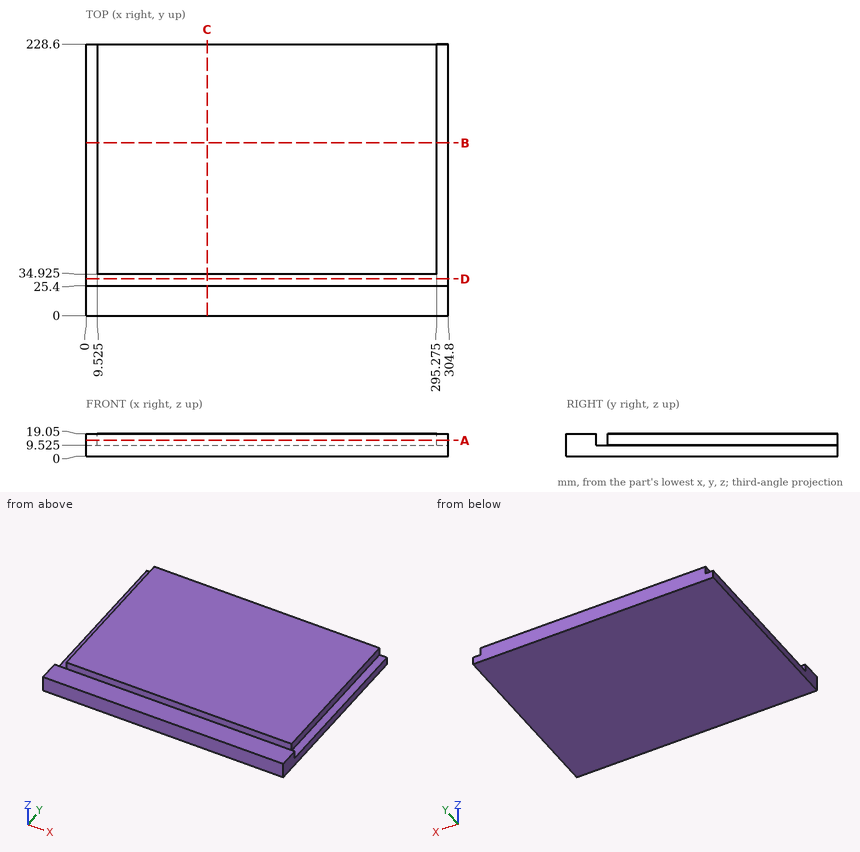
Verification items for this drawing (mm, ordinates from the low corner). Coordinates: 2 decimals unless noted, no trailing zeros. Order: outer loops, then holes, each group sorted by start corner. A loop starts at its lowest first (then second) coordinate and runs counter-clockwise, first axis right, second up. Notation, with made-up numbers: (-29, 44.25) -> (-4, 44.25) arc R23 cw to (-4, 74.25) -> close; hole circle Ø6 at (63, 82.25). An arc over 180 degrees is marked (long way). Put each result on its own line as item: value. Start each with the question number.
1. Cross-section at A-A, the plane z = 13.5. Record the boundary of the cut face in (x, y) (3 decimals).
2. Cross-section at B-B, the plane y = 145.5. Record the boundary of the cut face in (x, z) (3 decimals), then the cut area to 4 significant figures.
3. Cross-section at C-C, the plane x = 102. Record the boundary of the cut face in (y, z) (3 decimals), then the cut area to 3 significant figures.
4. Go/stop test with flat-tipped pins: pin 1 Ø5 at (y, z) = (91, 16) entering from +X (3 decimals); pin 2 Ø4 at (y, z) = (96.5, 13) entering from -X (3 decimals). Record where each tip stops, or that it passes through.
5. Cross-section at D-D, the plane y = 31. Record the boundary of the cut face in (x, z) (3 decimals), then the cut area to 3 significant figures.
6. Material ranges on L1, parallel to Y at x = 143.5, z = 15 (3 decimals); L2, parallel to X at y = 38, z = 15.25 (3 decimals); L3, parallel to Z at x = 137.5, y = 29.5 (3 decimals), recorded low to high. Write a range as [from, to].
Computed:
1. outline: (0, 0) -> (304.8, 0) -> (304.8, 25.4) -> (0, 25.4) -> close; (9.525, 34.925) -> (295.275, 34.925) -> (295.275, 228.6) -> (9.525, 228.6) -> close
2. outline: (0, 0) -> (304.8, 0) -> (304.8, 9.525) -> (295.275, 9.525) -> (295.275, 19.05) -> (9.525, 19.05) -> (9.525, 9.525) -> (0, 9.525) -> close
2. area: 5,625 mm2
3. outline: (0, 0) -> (228.6, 0) -> (228.6, 19.05) -> (34.925, 19.05) -> (34.925, 9.525) -> (25.4, 9.525) -> (25.4, 19.05) -> (0, 19.05) -> close
3. area: 4,260 mm2
4. pin 1: x = 295.275
4. pin 2: x = 9.525
5. outline: (0, 0) -> (304.8, 0) -> (304.8, 9.525) -> (0, 9.525) -> close
5. area: 2,900 mm2
6. L1: [0, 25.4], [34.925, 228.6]
6. L2: [9.525, 295.275]
6. L3: [0, 9.525]
